Here's how the part is built. I have some questions about the finished solid (model axes, mm). A direction names the side the tool comes from. Give positions to 0.01 mm unless a question says otherwise; leave off trailing zeros. Loops run counter-clockwise (first coordinate to the right, second up) from the corner with the lowest first, then second, coordinate; pieces in that order, holes last. Notation, with made-up numbers: (61.5, 6.25) -> (106.5, 6.25) arc R14 cw to (106.5, 29.25) -> close; hole circle Ø9 at (-18, -12). An arc over 180 degrees is marked (long way). Answer in a Markdown table with one row per item. Add a question column.
Item 1: We'd pull the mould along Y, two halves only. Please class faces 4 (the face through (40.343, -9.128, 1.014)), 5 (the face through (28.978, 13.034, 0.986)), 6 (the face through (-14.91, 16.77, 1.01)): released by +Y, released by -Y, zero draft, split by the parting line, or undercut.
Item 2: If we section it at C-C (y = 8.5): Write out the boundary of the cut face in (x, z).
Item 3: If I drill on line 1 (Y direction, x = 50, z = 1.35); line 2 (Y direction, x = 7.5, z = 1.3); line 3 (X direction, y = -9, z = 1.5), over which ranges is the centre line in solid material (lowest first)?
Item 4: If we section it at B-B (y = 0): Write out the boundary of the cut face in (x, z).
Item 5: If we section it at A-A (x = 7.5): Write out the boundary of the cut face in (y, z), then the cut area to 3 significant figures.
Item 6: For P1, Ø3, axis at x = -12.5, y = 13.5, coming from the +Z side; P2, Ø1.5, axis at x = -31, y = 1, coming from the -Z side; P3, Ø0.6, axis at x = 15.5, z = 0.5, coming from the -Y side, each with a flat end and sliding along its axis, tell me the tip position at first contact or that it passes through.
Item 7: If we section it at D-D (z = 1.3): Give the number of separate pieces and of enclosed holes in the cut face, then the cut area to 3 significant figures.
Item 8: Which directions (+Z, -Z, +X, -X, +Y, -Y) give clear straight access to the entire face, cutting with the end or side of a thin tool? Please do faces 1 (the face through (16, -6.963, 1)), 2 (the face through (61.283, -1.229, 0.986)), 3 (the face through (-37, 11.35, 1)).
Autodesk Inventor part; units mm, degrees
ref_plane "YZ Plane" through (0, 0, 0) normal (1, 0, 0) x (0, 1, 0)
ref_plane "XZ Plane" through (0, 0, 0) normal (0, 1, 0) x (-1, 0, 0)
ref_plane "XY Plane" through (0, 0, 0) normal (0, 0, 1) x (1, 0, 0)
sketch "スケッチ1" plane through (0, 0, 0) normal (0, 0, 1) x (1, 0, 0)
  line L0 (-50, 0) -> (50, 0) construction
  circle A0 centre (-50, 0) radius 4
  circle A1 centre (50, 0) radius 6
  line L1 (-50, 11.35) -> (-23, 11.35)
  line L2 (-50, -11.35) -> (50, -11.35)
  arc A2 (50, -11.35) -> (50, 11.35) centre (50, 0) ccw
  line L3 (30, 17) -> (-15, 17)
  line L4 (-15, 17) -> (-23, 11.35)
  line L5 (-24.9115, 10) -> (41.8474, 10) construction
  line L6 (-15, 17) -> (-15, 10) construction
  line L7 (30, 17) -> (30, 10) construction
  circle A3 centre (27.5, 13.5) radius 1.55
  circle A4 centre (-12.5, 13.5) radius 1.55
  circle A5 centre (7.5, 13.5) radius 1.55
  line L8 (-15, 13.5) -> (30, 13.5) construction
  line L9 (30, 16) -> (-15, 16) construction
  line L10 (-15, 16) -> (-15, 11) construction
  line L11 (-15, 11) -> (30, 11) construction
  line L12 (30, 11) -> (30, 16) construction
  line L13 (-23, 11.35) -> (50, 11.35)
  arc A6 (-50, 11.35) -> (-50, -11.35) centre (-50, 0) ccw
  line L14 (7.5, 17) -> (7.5, 10.5172) construction
  line L15 (30, 17) -> (52.8887, 10.9762)
  point P0 (0, 0)
  point P1 (0, 0)
  point P2 (55.7736, 9.7718)
  point P3 (38, 11.35)
  dimension "d0" = 100
  dimension "d1" = 8
  dimension "d8" = 12
  dimension "d10" = 7
  dimension "d11" = 45
  dimension "d12" = 2.5
  dimension "d13" = 3.1
  dimension "d14" = 2.5
  dimension "d15" = 20
  dimension "d17" = 5
  dimension "d18" = 11
  dimension "d69" = 11.35
  dimension "d72" = 11.35
  dimension "d87" = 8
  dimension "d88" = 8
extrude "押し出し1" add sketch "スケッチ1" along normal blind 2
fillet "フィレット1" radius 5 4 edges at (-23, 11.35, 1) (-15, 17, 1) (30, 17, 1) (-50, 11.35, 1)
sketch "スケッチ2" plane through (0, 0, 2) normal (0, 0, 1) x (1, 0, 0)
  arc A0 (50, -11.35) -> (52.8887, 10.9762) centre (50, 0) ccw
  line L0 (18, -20) -> (-35.4549, -20) construction
  line L1 (-76.9372, -11.5) -> (-72, -11.5)
  line L2 (-76.9372, -12.4) -> (-76.9372, -11.5)
  line L3 (-71.9872, -11.45) -> (-76.9872, -11.45)
  line L4 (-76.9872, -11.45) -> (-76.9872, -12.45)
  circle A1 centre (-50, 0) radius 4
  circle A2 centre (-50, 0) radius 5.5 construction
  circle A3 centre (50, 0) radius 6
  line L5 (83.3205, -17.7128) -> (50, 0) construction
  line L6 (50, 0) -> (18, -20) construction
  line L7 (83.3205, -17.7128) -> (37.8533, -17.7128) construction
  line L8 (-13.4166, -12.4128) -> (46.4577, -12.4128)
  line L9 (46.4577, -12.4128) -> (46.4577, -11.5128)
  line L10 (46.4577, -11.5128) -> (45.5205, -11.5128)
  line L11 (45.5205, -11.5128) -> (35.5205, -7.0128)
  line L12 (35.5205, -7.0128) -> (-2.4795, -7.0128)
  line L13 (-2.4795, -7.0128) -> (-12.4795, -11.5128)
  line L14 (-12.4795, -11.5128) -> (-13.4166, -11.5128)
  line L15 (-13.4166, -11.5128) -> (-13.4166, -12.4128)
  line L16 (-12.4902, -11.4628) -> (-2.4902, -6.9628)
  line L17 (-2.4902, -6.9628) -> (35.5312, -6.9628)
  line L18 (35.5312, -6.9628) -> (45.5312, -11.4628)
  line L19 (45.5312, -11.4628) -> (46.5077, -11.4628)
  line L20 (46.5077, -11.4628) -> (46.5077, -12.4628)
  line L21 (46.5077, -12.4628) -> (-13.4666, -12.4628)
  line L22 (-13.4666, -12.4628) -> (-13.4666, -11.4628)
  line L23 (-13.4666, -11.4628) -> (-12.4902, -11.4628)
  point P0 (56.6914, 9.1677)
  point P1 (0, 0)
  point P2 (50, 11.35)
  dimension "d19" = 20
  dimension "d20" = 32
  dimension "d32" = 11
  dimension "d33" = 120
  dimension "d37" = 37.8
  dimension "d38" = 6.2
  dimension "d39" = 0.05
  dimension "d49" = 38
  dimension "d50" = 10
  dimension "d51" = 10
  dimension "d52" = 4.5
  dimension "d53" = 0.9
  dimension "d54" = 59.9743
extrude "押し出し2" cut sketch "スケッチ2" against normal blind 10 contours L15 L14 L13 L12 L11 L10 L9 L8 | L16 L17 L18 L19 L20 L21 L22 L23
fillet "フィレット2" radius 2 4 edges at (45.2805, -11.35, 1) (-12.2395, -11.35, 1) (35.5312, -6.9628, 1) (-2.4902, -6.9628, 1)
sketch "スケッチ4" plane through (0, 0, 2) normal (0, 0, 1) x (1, 0, 0)
  circle A0 centre (50, 0) radius 6
  circle A1 centre (50, 0) radius 8.5 construction
  line L0 (50, 0) -> (50, 8.5) construction
  circle A2 centre (50, 8.5) radius 1.35
  circle A3 centre (41.5, 0) radius 1.35
  circle A4 centre (50, -8.5) radius 1.35
  circle A5 centre (58.5, 0) radius 1.35
  point P0 (0, 0)
  dimension "d61" = 17
  dimension "d62" = 2.7
  dimension "d65" = 360
extrude "押し出し4" cut sketch "スケッチ4" against normal through all contours A2 | A3 | A4 | A5
sketch "スケッチ6" plane through (0, 0, 2) normal (0, 0, 1) x (1, 0, 0)
  circle A0 centre (-50, 0) radius 4
  circle A1 centre (-50, 0) radius 8.5 construction
  circle A2 centre (-58.5, 0) radius 2.5
  line L0 (-50, 0) -> (-58.5, 0) construction
  line L1 (-50, 0) -> (-41.5, 0) construction
  circle A3 centre (-41.5, 0) radius 2.5
  arc A4 (-50, 11.35) -> (-50, -11.35) centre (-50, 0) ccw
  line L2 (-58.5, -2.5) -> (-61.0712, -2.5)
  line L3 (-58.5, 2.5) -> (-61.0712, 2.5)
  point P0 (0, 0)
  dimension "d78" = 17
  dimension "d79" = 5
  dimension "d82" = 360
extrude "押し出し6" cut sketch "スケッチ6" against normal through all contours A2 | A2 L2 A4 L3 | A3
fillet "フィレット4" radius 2 2 edges at (-61.0712, 2.5, 1) (-61.0712, -2.5, 1)
equation "\"d14\" = d12"
properties part number "リンク_メインフレーム_6_4" material "GFRP"
Recorded:
| question | item | result |
|---|---|---|
| 1 | face 4 | released by -Y |
| 1 | face 5 | undercut |
| 1 | face 6 | released by +Y |
| 2 | outline | (-57.52, 0) -> (48.65, 0) -> (48.65, 2) -> (-57.52, 2) -> close; (51.35, 0) -> (57.52, 0) -> (57.52, 2) -> (51.35, 2) -> close |
| 3 | line 1 | y = -11.35 to -9.85, -7.15 to -6, 6 to 7.15, 9.85 to 11.74 |
| 3 | line 2 | y = -6.96 to 11.95, 15.05 to 17 |
| 3 | line 3 | x = -56.92 to -7.02, 40.06 to 48.75, 51.25 to 56.92 |
| 4 | outline | (-56, 0) -> (-54, 0) -> (-54, 2) -> (-56, 2) -> close; (-46, 0) -> (-44, 0) -> (-44, 2) -> (-46, 2) -> close; (-39, 0) -> (40.15, 0) -> (40.15, 2) -> (-39, 2) -> close; (42.85, 0) -> (44, 0) -> (44, 2) -> (42.85, 2) -> close; (56, 0) -> (57.15, 0) -> (57.15, 2) -> (56, 2) -> close; (59.85, 0) -> (61.35, 0) -> (61.35, 2) -> (59.85, 2) -> close |
| 5 | outline | (-6.96, 0) -> (11.95, 0) -> (11.95, 2) -> (-6.96, 2) -> close; (15.05, 0) -> (17, 0) -> (17, 2) -> (15.05, 2) -> close |
| 5 | area | 41.7 mm^2 |
| 6 | P1 | passes through |
| 6 | P2 | stops at z = 0 |
| 6 | P3 | stops at y = -6.96 |
| 7 | separate pieces | 1 |
| 7 | enclosed holes | 10 |
| 7 | area | 2,550 mm^2 |
| 8 | face 1 | +Z, -Z, -Y |
| 8 | face 2 | +Z, -Z, +X |
| 8 | face 3 | +Z, -Z, -X, +Y |
